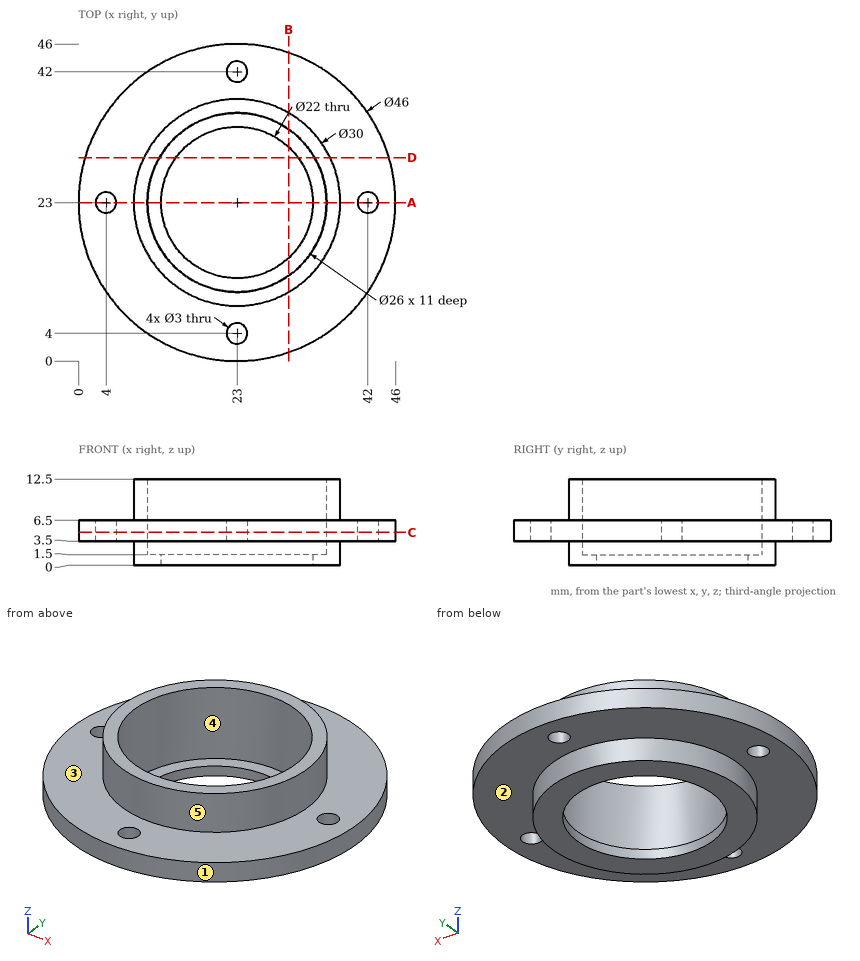
Input: dimensioned drawing with shaded views. Units: mm. Origin: part minimum x, y, z. A direction names the side the tool comes from. Give positions to 0.01 mm unless a question says otherwise; leave off trailing zeros. Write each loop counter-clockwise with the first axis right and the second up, starting at its lowest first coordinate (ties: lowest second). Pieces come first, ordered by that corner, then holes. Notation, with made-up numbers: (-17, 39.25) -> (-11, 39.25) arc R18 cw to (-11, 62.25) -> close; hole circle Ø3 at (73.5, 57). An arc over 180 degrees is marked (long way). Answer as a JSON object with one key per item and string values.
1. Cut plane C-C on z = 4.75. Output: boundary loops of the cut face in (x, y), and give its area (3 significant figures).
Ans:
{"outline": "circle Ø46 at (23, 23); hole circle Ø3 at (4, 23); hole circle Ø26 at (23, 23); hole circle Ø3 at (23, 4); hole circle Ø3 at (23, 42); hole circle Ø3 at (42, 23)", "area": "1,100 mm^2"}
2. Cut plane D-D on y = 29.5. Output: boundary loops of the cut face in (x, z), and give its area (3 significant figures).
Ans:
{"outline": "(0.94, 3.5) -> (9.48, 3.5) -> (9.48, 0) -> (14.13, 0) -> (14.13, 1.5) -> (11.74, 1.5) -> (11.74, 12.5) -> (9.48, 12.5) -> (9.48, 6.5) -> (0.94, 6.5) -> close; (31.87, 0) -> (36.52, 0) -> (36.52, 3.5) -> (45.06, 3.5) -> (45.06, 6.5) -> (36.52, 6.5) -> (36.52, 12.5) -> (34.26, 12.5) -> (34.26, 1.5) -> (31.87, 1.5) -> close", "area": "115 mm^2"}
3. Cut plane B-B on x = 30.5. Output: boundary loops of the cut face in (y, z), and give its area (3 significant figures).
Ans:
{"outline": "(1.26, 3.5) -> (10.01, 3.5) -> (10.01, 0) -> (14.95, 0) -> (14.95, 1.5) -> (12.38, 1.5) -> (12.38, 12.5) -> (10.01, 12.5) -> (10.01, 6.5) -> (1.26, 6.5) -> close; (31.05, 0) -> (35.99, 0) -> (35.99, 3.5) -> (44.74, 3.5) -> (44.74, 6.5) -> (35.99, 6.5) -> (35.99, 12.5) -> (33.62, 12.5) -> (33.62, 1.5) -> (31.05, 1.5) -> close", "area": "120 mm^2"}
4. Ray query, probe 1 along Y at (x, z) = (23, 4.5); probe 2 along Y at (x, z) = (22.5, 2.5); probe 3 along Y at (x, z) = (25.5, 7.25). Return the intervals inside material, ascending. Write a range as from..to.
Ans:
{"probe 1": "y = 0..2.5, 5.5..10, 36..40.5, 43.5..46", "probe 2": "y = 8.01..10.01, 35.99..37.99", "probe 3": "y = 8.21..10.24, 35.76..37.79"}
5. Cut plane A-A on y = 23. Output: boundary loops of the cut face in (x, z), and give its area (3 significant figures).
Ans:
{"outline": "(0, 3.5) -> (2.5, 3.5) -> (2.5, 6.5) -> (0, 6.5) -> close; (5.5, 3.5) -> (8, 3.5) -> (8, 0) -> (12, 0) -> (12, 1.5) -> (10, 1.5) -> (10, 12.5) -> (8, 12.5) -> (8, 6.5) -> (5.5, 6.5) -> close; (34, 0) -> (38, 0) -> (38, 3.5) -> (40.5, 3.5) -> (40.5, 6.5) -> (38, 6.5) -> (38, 12.5) -> (36, 12.5) -> (36, 1.5) -> (34, 1.5) -> close; (43.5, 3.5) -> (46, 3.5) -> (46, 6.5) -> (43.5, 6.5) -> close", "area": "86.0 mm^2"}
6. Mould query, pull axis Y, two halves, no side actions, for the marked faces 3, 4 and 5. Classes: pulls with the +Y half, pulls with the -Y half, needs draft (parallel to the pull), parting line crosses it, or undercut.
Ans:
{"face 3": "needs draft", "face 4": "undercut", "face 5": "parting line crosses it"}
7. Contact query for flat-ended pins moving along their axis: pin 1 (1.5 mm diameter, centred on y = 23, z = 11, fed in from -X); pin 2 (4 mm diameter, centred on x = 23, y = 4, fed in from +Z); pin 3 (3 mm diameter, centred on x = 19, z = 6.5, fed in from -Y). Output: stop coordinate, or through.
Ans:
{"pin 1": "stops at x = 8", "pin 2": "stops at z = 6.5", "pin 3": "stops at y = 0.14"}
8. Access query for the marked faces 1 and 2. Directions: +Z, -Z, +X, -X, +Y, -Y. A direction counts if a zero-diameter tool reaches every point of the face in a straight line with its end or side. Return the directions, or none.
Ans:
{"face 1": "+Z, -Z", "face 2": "-Z"}
